```python
from build123d import *

# Parameters (mm, degrees)
BOSS_EXTRUDE1_DEPTH      = 10.16
BOSS_EXTRUDE1_DEPTH_BACK = 10.16
SKETCH4_R                = 25.4
SKETCH5_R                = 2.54
BOSS_EXTRUDE2_DEPTH      = 2.54
FILLET1_R                = 2.54


with BuildPart() as part:
    # Sketch1 → Revolve1 (revolve)
    with BuildSketch(Plane(origin=(0, 0, 0), x_dir=(0, 0, -1), z_dir=(1, 0, 0)), mode=Mode.PRIVATE) as revolve1_sk:
        with BuildLine():
            Line((-12.7, 25.4), (12.7, 25.4))
            ThreePointArc((12.7, 25.4), (0, 38.1), (-12.7, 25.4))
        make_face()
    revolve(revolve1_sk.sketch.rotate(Axis((0, 0, 0), (0, 0, -1)), 90), axis=Axis((0, 0, 0), (0, 0, -1)))

    # Sketch4 → Boss-Extrude1 (add, two sides: drawn at the far end of the back side and taken through both)
    with BuildSketch(Plane.XY.offset(-BOSS_EXTRUDE1_DEPTH_BACK)):
        Circle(SKETCH4_R)
    extrude(amount=BOSS_EXTRUDE1_DEPTH + BOSS_EXTRUDE1_DEPTH_BACK)

    # Sketch5 → Boss-Extrude2 (add)
    with BuildSketch(Plane.XY.offset(10.16)):
        Circle(SKETCH5_R)
    boss_extrude2 = extrude(amount=BOSS_EXTRUDE2_DEPTH)

    # Mirror1: Boss-Extrude2 across plane
    add(boss_extrude2.mirror(Plane.XY))

    # Fillet1
    # the kernel refuses this fillet: 2.54 mm, written as the material it takes off along each edge
    with BuildSketch(Plane(origin=(0, 0, -12.7), x_dir=(1, 0, 0), z_dir=(0, 1, 0))) as fillet1_piece_1:
        with BuildLine():
            CenterArc((27.920078124, -2.8575), FILLET1_R, 75.638488437, 97.180755781)
            Line((25.4, -2.54), (25.349598438, -2.53365))
            ThreePointArc((25.349598438, -2.53365), (25.3492, -1.27), (25.3492, 0))
            Line((25.3492, 0), (25.4, 0.0508))
            ThreePointArc((25.4, 0.0508), (26.99385, -0.049207819), (28.562698045, -0.3476625))
            Line((28.562698045, -0.3476625), (28.550097655, -0.396875))
        make_face()
    revolve(axis=Axis((0, 0, -12.7), (0, 0, -1)), mode=Mode.SUBTRACT)
    with BuildSketch(Plane(origin=(0, 0, 12.7), x_dir=(1, 0, 0), z_dir=(0, 1, 0))) as fillet1_piece_2:
        with BuildLine():
            CenterArc((27.920078124, 2.8575), FILLET1_R, 187.180755781, 97.180755781)
            Line((28.550097655, 0.396875), (28.562698045, 0.3476625))
            ThreePointArc((28.562698045, 0.3476625), (26.99385, 0.049207819), (25.4, -0.0508))
            Line((25.4, -0.0508), (25.3492, 0))
            ThreePointArc((25.3492, 0), (25.3492, 1.27), (25.349598438, 2.53365))
            Line((25.349598438, 2.53365), (25.4, 2.54))
        make_face()
    revolve(axis=Axis((0, 0, 12.7), (0, 0, -1)), mode=Mode.SUBTRACT)


solid = part.part
```
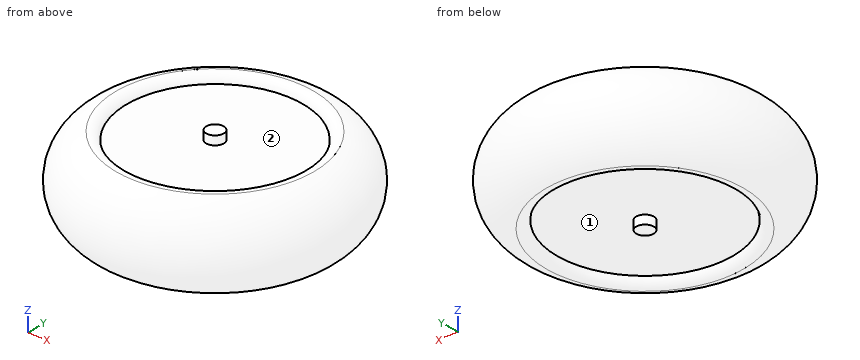
Geometry: final body of the model. Coordinates: model frame, mm. Face numbers are marked on the shaded views. Round coordinates to 2 decimals unless told otherwise and drop trailing zeros. Order: outer loops, then holes, each group sorted by start corner. A loop starts at its lowest first (then second) coordinate and runs counter-clockwise, first axis right, second up. Notation, with made-up numbers: (-32, 61.5) -> (3, 61.5) arc R25 ccw to (3, 73.5) -> close; hole circle Ø1 at (62.25, 71). An arc over 180 degrees is marked (long way). Use one line per item in the form item = value. Start each with the question number.
1. Cut plane D-D (z = -4.25). Return the cut outline in (x, y), then the cut area to 3 significant figures.
2. Draft query along Y for the marked faces 1 and 2. Return one class per face: pulls with the +Y half, pulls with the -Y half, needs draft (parallel to the pull), parting line crosses it, or undercut.
3. Cut plane C-C (z = 1.25). Return the cut outline in (x, y).
4. Line query: probe 1 along Z at (x, y) = (0, -8); probe 2 along X at (y, z) = (-13, 5.5); probe 3 along Z at (x, y) = (-32, -10). Output: solid intervals per line, ascending.
5. Cut plane A-A (x = 0). Return the cut outline in (y, z).
6. Pin query (flat end, axial travel): pin 1 Ø1.5 at (x, z) = (-12, -3) entering from -Y; pin 2 Ø6 at (x, z) = (-18.5, -8.5) entering from -Y; pin 3 Ø12 at (y, z) = (-18.5, -3.5) entering from -X. Return the tip coordinate at first contact, or that it passes through.
Solution:
q1.outline = circle Ø74.74 at (0, 0)
q1.area = 4,390 mm^2
q2.face_1 = undercut
q2.face_2 = undercut
q3.outline = circle Ø76.08 at (0, 0)
q4.probe_1 = -10.16 to 10.16
q4.probe_2 = -34.48 to 34.48
q4.probe_3 = -9.76 to 9.76
q5.outline = (-28.55, -12.3) arc R2.54 ccw to (-25.4, -10.16) -> (-2.54, -10.16) -> (-2.54, -12.7) -> (2.54, -12.7) -> (2.54, -10.16) -> (25.4, -10.16) arc R2.54 ccw to (28.55, -12.3) arc R12.7 ccw to (28.55, 12.3) arc R2.54 ccw to (25.4, 10.16) -> (2.54, 10.16) -> (2.54, 12.7) -> (-2.54, 12.7) -> (-2.54, 10.16) -> (-25.4, 10.16) arc R2.54 ccw to (-28.55, 12.3) arc R12.7 ccw to start
q6.pin_1 = -36.08
q6.pin_2 = -32.5
q6.pin_3 = -35.78
